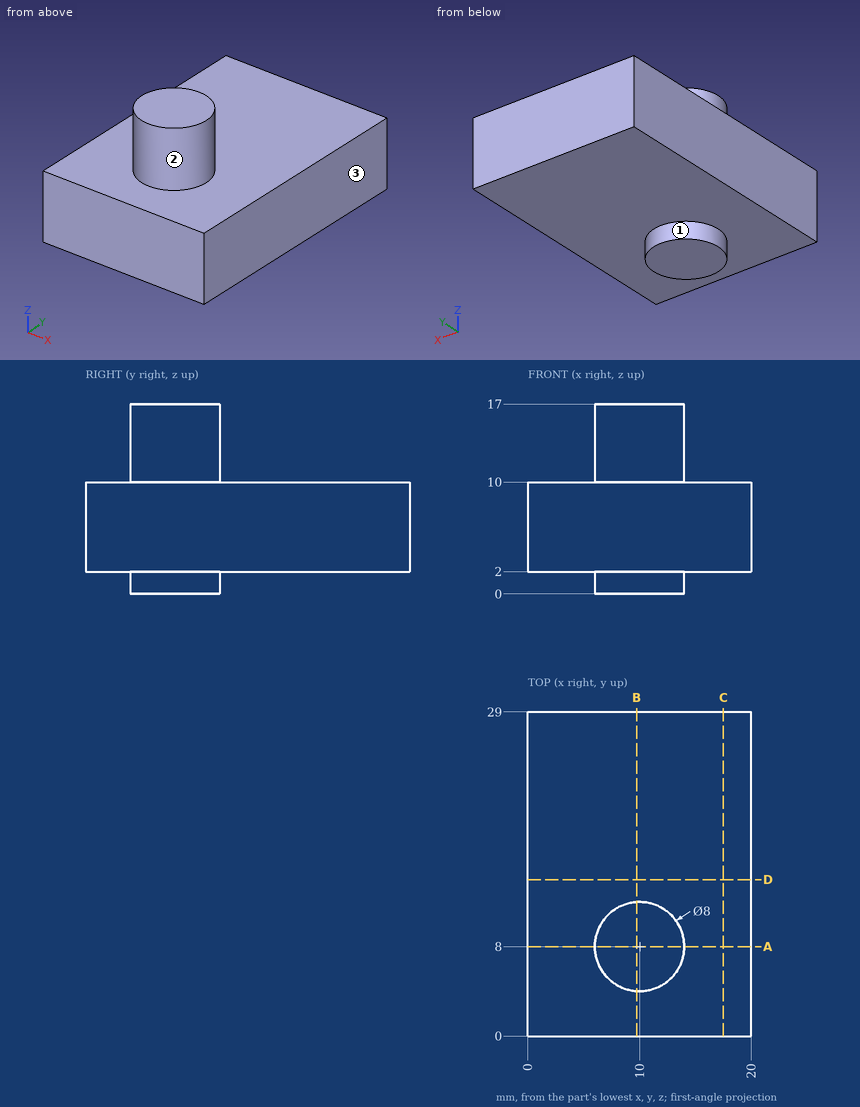
For this review, use the dimensioned drawing (mm, ordinates from the lowest corner) and the shaded views. A direction names the side the tool comes from. Give positions to 0.01 mm unless a question says otherwise; leave off trailing zeros. Order: outer loops, then holes, each group sorted by start corner. A loop starts at its lowest first (then second) coordinate and runs counter-clockwise, first axis right, second up. Notation, with made-up numbers: (-15, -6.75) - (21, -6.75) arc R30 ccw to (21, 26.25) - close; hole circle Ø6 at (22.5, 81). An arc over 180 degrees is marked (long way). Write item = value, one per line. Start each with the question number.
Q1. To check wall thickness, follow L1, parallel to Z at x = 12, y = 16. State the ranges of the line that lie inside material, in increasing order. Write a range as from..to.
Q2. We need section C-C on x = 17.5. State the section outline as (y, z) points.
Q3. We need section D-D on y = 14. State the section outline as (x, z) points.
Q4. We need section B-B on x = 9.75. State the section outline as (y, z) points, plus the area to 3 significant figures.
Q5. Tool access review of the marked faces 1, 2 and 3: name each direction out of +Z, -Z, +X, -X, +Y, -Y from which nothing blocks a thin tool from reaching the whole face with its end or side.
Q6. Clearance check with flat-ended pins moving along their axes: pin 1 Ø1.5 at (y, z) = (6.5, 12) entering from +X; pin 2 Ø3 at (x, y) = (2.5, 3.5) entering from -Z. State where each tip first meets the part, or that it passes through.
Q7. We need section A-A on y = 8. State the section outline as (x, z) points.
Working result:
q1.L1 = 2..10
q2.outline = (0, 2) - (29, 2) - (29, 10) - (0, 10) - close
q3.outline = (0, 2) - (20, 2) - (20, 10) - (0, 10) - close
q4.outline = (0, 2) - (4.01, 2) - (4.01, 0) - (11.99, 0) - (11.99, 2) - (29, 2) - (29, 10) - (11.99, 10) - (11.99, 17) - (4.01, 17) - (4.01, 10) - (0, 10) - close
q4.area = 304 mm²
q5.face_1 = -Z
q5.face_2 = +Z
q5.face_3 = +Z, -Z, +X, +Y, -Y
q6.pin_1 = 13.93
q6.pin_2 = 2
q7.outline = (0, 2) - (6, 2) - (6, 0) - (14, 0) - (14, 2) - (20, 2) - (20, 10) - (14, 10) - (14, 17) - (6, 17) - (6, 10) - (0, 10) - close
